```python
from build123d import *

# Parameters (mm, degrees)
SKIZZE1_W                                            = 80
SKIZZE1_H                                            = 120
AUFSATZ_LINEAR_AUSTRAGEN1_DEPTH                      = 5
FORMSENKUNG_F_R_M4_SENKSCHRAUBE_MIT_INNE_D           = 4.3
FORMSENKUNG_F_R_M4_SENKSCHRAUBE_MIT_INNE_DEPTH       = 11.5
FORMSENKUNG_F_R_M4_SENKSCHRAUBE_MIT_INNE_CSINK_D     = 9.18
FORMSENKUNG_F_R_M4_SENKSCHRAUBE_MIT_INNE_CSINK_ANGLE = 90
FORMSENKUNG_F_R_M4_SENKSCHRAUBE_MIT_INNE_TIP         = 1.291850331
F_3_0MM_STIFTLOCH1_D                                 = 3
F_3_0MM_STIFTLOCH1_DEPTH                             = 11.5
F_3_0MM_STIFTLOCH1_TIP                               = 0.901290929
STIRNSENKUNG_F_R_M3_FLACHKOPFSCHRAUB_2_COUNT         = 2
STIRNSENKUNG_F_R_M3_FLACHKOPFSCHRAUB_2_PITCH         = 15
STIRNSENKUNG_F_R_M3_FLACHKOPFSCHRAUB_3_COUNT         = 2
STIRNSENKUNG_F_R_M3_FLACHKOPFSCHRAUB_3_PITCH         = 25
STIRNSENKUNG_F_R_M3_FLACHKOPFSCHRAUB_4_COUNT         = 2
STIRNSENKUNG_F_R_M3_FLACHKOPFSCHRAUB_4_PITCH         = 20
STIRNSENKUNG_F_R_M3_FLACHKOPFSCHRAUB_5_COUNT         = 2
STIRNSENKUNG_F_R_M3_FLACHKOPFSCHRAUB_5_PITCH         = 90
STIRNSENKUNG_F_R_M3_FLACHKOPFSCHRAUB_6_COUNT         = 2
STIRNSENKUNG_F_R_M3_FLACHKOPFSCHRAUB_6_PITCH         = 105
STIRNSENKUNG_F_R_M3_FLACHKOPFSCHRAUB_7_COUNT         = 2
STIRNSENKUNG_F_R_M3_FLACHKOPFSCHRAUB_7_PITCH         = 106.887791632
STIRNSENKUNG_F_R_M3_FLACHKOPFSCHRAUB_8_COUNT         = 2
STIRNSENKUNG_F_R_M3_FLACHKOPFSCHRAUB_8_PITCH         = 92.195444573
M10_GEWINDEBOHRUNG1_D                                = 8.5
LINEARES_MUSTER1_COUNT                               = 2
LINEARES_MUSTER1_PITCH                               = 50


with BuildPart() as part:
    # Skizze1 → Aufsatz-Linear austragen1 (new body)
    with BuildSketch(Plane.XY.offset(10)):
        with Locations((-40, 60)):
            Rectangle(SKIZZE1_W, SKIZZE1_H)
    extrude(amount=-AUFSATZ_LINEAR_AUSTRAGEN1_DEPTH)

    # Formsenkung für M4 Senkschraube mit Innensechskant1
    with Locations(Plane.XY.offset(10)):
        with Locations((-56, 60), (-25, 60)):
            CounterSinkHole(FORMSENKUNG_F_R_M4_SENKSCHRAUBE_MIT_INNE_D / 2, FORMSENKUNG_F_R_M4_SENKSCHRAUBE_MIT_INNE_CSINK_D / 2, depth=FORMSENKUNG_F_R_M4_SENKSCHRAUBE_MIT_INNE_DEPTH, counter_sink_angle=FORMSENKUNG_F_R_M4_SENKSCHRAUBE_MIT_INNE_CSINK_ANGLE)
            with Locations((0, 0, -(FORMSENKUNG_F_R_M4_SENKSCHRAUBE_MIT_INNE_DEPTH + FORMSENKUNG_F_R_M4_SENKSCHRAUBE_MIT_INNE_TIP / 2))):  # 118° drill point
                Cone(0, FORMSENKUNG_F_R_M4_SENKSCHRAUBE_MIT_INNE_D / 2, FORMSENKUNG_F_R_M4_SENKSCHRAUBE_MIT_INNE_TIP, mode=Mode.SUBTRACT)

    # Ø3.0mm Stiftloch1
    with Locations(Plane.XY.offset(10)):
        with Locations((-56, 74), (-25, 74), (-25, 46), (-56, 46)):
            Hole(F_3_0MM_STIFTLOCH1_D / 2, depth=F_3_0MM_STIFTLOCH1_DEPTH)
            with Locations((0, 0, -(F_3_0MM_STIFTLOCH1_DEPTH + F_3_0MM_STIFTLOCH1_TIP / 2))):  # 118° drill point
                Cone(0, F_3_0MM_STIFTLOCH1_D / 2, F_3_0MM_STIFTLOCH1_TIP, mode=Mode.SUBTRACT)

    # Skizze25 → Stirnsenkung für M3 Flachkopfschraube mit Schlitz2 (revolve, cut)
    with BuildSketch(Plane(origin=(-25, 112.5, 5), x_dir=(0, 1, 0), z_dir=(1, 0, 0))):
        Polygon((0, 0), (0, 9.521463052), (1.7, 8.5), (1.7, 2.4), (3.5, 2.4), (3.5, 0), align=None)
    stirnsenkung_f_r_m3_flachkopfschraube_mi = revolve(axis=Axis((-25, 112.5, -1.35), (0, 0, 1)), mode=Mode.SUBTRACT)

    # Stirnsenkung f_r M3 Flachkopfschraub 2: Stirnsenkung für M3 Flachkopfschraube mit Schlitz2 ×2
    with Locations(*[(0, -i * STIRNSENKUNG_F_R_M3_FLACHKOPFSCHRAUB_2_PITCH, 0) for i in range(1, STIRNSENKUNG_F_R_M3_FLACHKOPFSCHRAUB_2_COUNT)]):
        add(stirnsenkung_f_r_m3_flachkopfschraube_mi, mode=Mode.SUBTRACT)

    # Stirnsenkung f_r M3 Flachkopfschraub 3: Stirnsenkung für M3 Flachkopfschraube mit Schlitz2 ×2
    with Locations(*[Vector(0.8000000000000007, -0.5999999999999991, 0) * (i * STIRNSENKUNG_F_R_M3_FLACHKOPFSCHRAUB_3_PITCH) for i in range(1, STIRNSENKUNG_F_R_M3_FLACHKOPFSCHRAUB_3_COUNT)]):
        add(stirnsenkung_f_r_m3_flachkopfschraube_mi, mode=Mode.SUBTRACT)

    # Stirnsenkung f_r M3 Flachkopfschraub 4: Stirnsenkung für M3 Flachkopfschraube mit Schlitz2 ×2
    with Locations(*[(i * STIRNSENKUNG_F_R_M3_FLACHKOPFSCHRAUB_4_PITCH, 0, 0) for i in range(1, STIRNSENKUNG_F_R_M3_FLACHKOPFSCHRAUB_4_COUNT)]):
        add(stirnsenkung_f_r_m3_flachkopfschraube_mi, mode=Mode.SUBTRACT)

    # Stirnsenkung f_r M3 Flachkopfschraub 5: Stirnsenkung für M3 Flachkopfschraube mit Schlitz2 ×2
    with Locations(*[(0, -i * STIRNSENKUNG_F_R_M3_FLACHKOPFSCHRAUB_5_PITCH, 0) for i in range(1, STIRNSENKUNG_F_R_M3_FLACHKOPFSCHRAUB_5_COUNT)]):
        add(stirnsenkung_f_r_m3_flachkopfschraube_mi, mode=Mode.SUBTRACT)

    # Stirnsenkung f_r M3 Flachkopfschraub 6: Stirnsenkung für M3 Flachkopfschraube mit Schlitz2 ×2
    with Locations(*[(0, -i * STIRNSENKUNG_F_R_M3_FLACHKOPFSCHRAUB_6_PITCH, 0) for i in range(1, STIRNSENKUNG_F_R_M3_FLACHKOPFSCHRAUB_6_COUNT)]):
        add(stirnsenkung_f_r_m3_flachkopfschraube_mi, mode=Mode.SUBTRACT)

    # Stirnsenkung f_r M3 Flachkopfschraub 7: Stirnsenkung für M3 Flachkopfschraube mit Schlitz2 ×2
    with Locations(*[Vector(0.1871121078899952, -0.9823385664224747, 0) * (i * STIRNSENKUNG_F_R_M3_FLACHKOPFSCHRAUB_7_PITCH) for i in range(1, STIRNSENKUNG_F_R_M3_FLACHKOPFSCHRAUB_7_COUNT)]):
        add(stirnsenkung_f_r_m3_flachkopfschraube_mi, mode=Mode.SUBTRACT)

    # Stirnsenkung f_r M3 Flachkopfschraub 8: Stirnsenkung für M3 Flachkopfschraube mit Schlitz2 ×2
    with Locations(*[Vector(0.2169304578186558, -0.9761870601839528, 0) * (i * STIRNSENKUNG_F_R_M3_FLACHKOPFSCHRAUB_8_PITCH) for i in range(1, STIRNSENKUNG_F_R_M3_FLACHKOPFSCHRAUB_8_COUNT)]):
        add(stirnsenkung_f_r_m3_flachkopfschraube_mi, mode=Mode.SUBTRACT)

    # M10 Gewindebohrung1 (through all)
    with Locations(Plane(origin=(0, 0, 5), x_dir=(-1, 0, 0), z_dir=(0, 0, -1))):
        with Locations((40, 15)):
            m10_gewindebohrung1 = Hole(M10_GEWINDEBOHRUNG1_D / 2)

    # Lineares Muster1: Stirnsenkung für M3 Flachkopfschraube mit Schlitz2 ×2
    with Locations(*[(-i * LINEARES_MUSTER1_PITCH, 0, 0) for i in range(1, LINEARES_MUSTER1_COUNT)]):
        add(stirnsenkung_f_r_m3_flachkopfschraube_mi, mode=Mode.SUBTRACT)

    # Lineares Muster1 copy 1 sketch → Lineares Muster1 copy 1 (revolve, cut)
    with BuildSketch(Plane(origin=(-75, 97.5, 5), x_dir=(0, 1, 0), z_dir=(1, 0, 0))):
        Polygon((0, 0), (0, 9.521463052), (1.7, 8.5), (1.7, 2.4), (3.5, 2.4), (3.5, 0), align=None)
    revolve(axis=Axis((-75, 97.5, -1.35), (0, 0, 1)), mode=Mode.SUBTRACT)

    # Lineares Muster1 copy 2 sketch → Lineares Muster1 copy 2 (revolve, cut)
    with BuildSketch(Plane(origin=(-55, 97.5, 5), x_dir=(0, 1, 0), z_dir=(1, 0, 0))):
        Polygon((0, 0), (0, 9.521463052), (1.7, 8.5), (1.7, 2.4), (3.5, 2.4), (3.5, 0), align=None)
    revolve(axis=Axis((-55, 97.5, -1.35), (0, 0, 1)), mode=Mode.SUBTRACT)

    # Lineares Muster1 copy 3 sketch → Lineares Muster1 copy 3 (revolve, cut)
    with BuildSketch(Plane(origin=(-55, 112.5, 5), x_dir=(0, 1, 0), z_dir=(1, 0, 0))):
        Polygon((0, 0), (0, 9.521463052), (1.7, 8.5), (1.7, 2.4), (3.5, 2.4), (3.5, 0), align=None)
    revolve(axis=Axis((-55, 112.5, -1.35), (0, 0, 1)), mode=Mode.SUBTRACT)

    # Lineares Muster1 copy 4 sketch → Lineares Muster1 copy 4 (revolve, cut)
    with BuildSketch(Plane(origin=(-75, 22.5, 5), x_dir=(0, 1, 0), z_dir=(1, 0, 0))):
        Polygon((0, 0), (0, 9.521463052), (1.7, 8.5), (1.7, 2.4), (3.5, 2.4), (3.5, 0), align=None)
    revolve(axis=Axis((-75, 22.5, -1.35), (0, 0, 1)), mode=Mode.SUBTRACT)

    # Lineares Muster1 copy 5 sketch → Lineares Muster1 copy 5 (revolve, cut)
    with BuildSketch(Plane(origin=(-75, 7.5, 5), x_dir=(0, 1, 0), z_dir=(1, 0, 0))):
        Polygon((0, 0), (0, 9.521463052), (1.7, 8.5), (1.7, 2.4), (3.5, 2.4), (3.5, 0), align=None)
    revolve(axis=Axis((-75, 7.5, -1.35), (0, 0, 1)), mode=Mode.SUBTRACT)

    # Lineares Muster1 copy 6 sketch → Lineares Muster1 copy 6 (revolve, cut)
    with BuildSketch(Plane(origin=(-55, 7.5, 5), x_dir=(0, 1, 0), z_dir=(1, 0, 0))):
        Polygon((0, 0), (0, 9.521463052), (1.7, 8.5), (1.7, 2.4), (3.5, 2.4), (3.5, 0), align=None)
    revolve(axis=Axis((-55, 7.5, -1.35), (0, 0, 1)), mode=Mode.SUBTRACT)

    # Lineares Muster1 copy 7 sketch → Lineares Muster1 copy 7 (revolve, cut)
    with BuildSketch(Plane(origin=(-55, 22.5, 5), x_dir=(0, 1, 0), z_dir=(1, 0, 0))):
        Polygon((0, 0), (0, 9.521463052), (1.7, 8.5), (1.7, 2.4), (3.5, 2.4), (3.5, 0), align=None)
    revolve(axis=Axis((-55, 22.5, -1.35), (0, 0, 1)), mode=Mode.SUBTRACT)

    # Spiegeln1: M10 Gewindebohrung1 across plane
    add(m10_gewindebohrung1.mirror(Plane(origin=(0, 60, 0), x_dir=(0, 0, 1), z_dir=(0, -1, 0))), mode=Mode.SUBTRACT)


solid = part.part
```
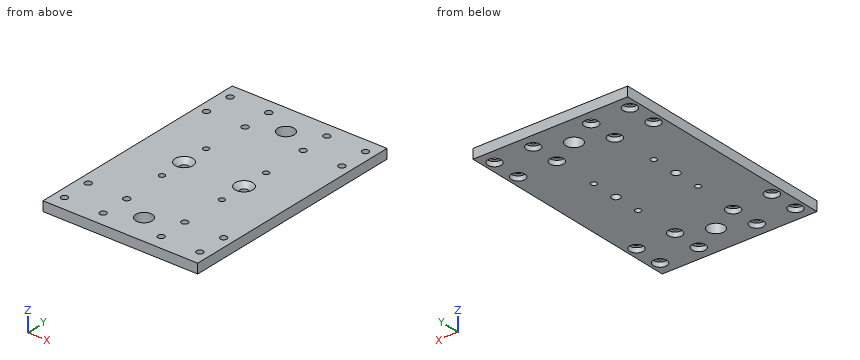
The model under review builds one solid part; all positions refer to its coordinate system, in mm. Round coordinates to 2 decimals unless told otherwise and drop trailing zeros. Write each loop counter-clockwise with the first axis right and the second up, starting at its lowest first coordinate (ties: lowest second). Pieces come first, ordered by that corner, then holes.
(1) We need section D-D on x = -40.5. Give the boundary of the cut face in (y, z).
(2) We need section A-A on y = 74. Give the boundary of the cut face in (x, z).
(3) We need section C-C on y = 105. Give the boundary of the cut face in (x, z), and give its area (4 significant figures).
(4) Insertion check: pin 1 (2.5 mm diameter, centred on x = -55, y = 97.5, fed in from +Z); pin 2 (5.5 mm diameter, centred on x = -25, y = 22.5, fed in from -Z). Each pin has a flat end and moves straight along its axis. Give the tip position at first contact, or say it passes through.
(5) Wall thickness on L1, parallel to Y at x = -75, z = 8.25; L2, parallel to X at y = 22.5, z = 6.2; L3, parallel to Y at x = -75, z = 5.95: over which ranges is each line inside the solid? List them lowest first.
(6) We need section B-B on z = 6.55. Give the number of separate pieces and of enclosed holes in the cut face, and give its area (3 significant figures).
Findings below:
1. outline: (0, 5) - (10.78, 5) - (10.78, 10) - (0, 10) - close; (19.22, 5) - (100.78, 5) - (100.78, 10) - (19.22, 10) - close; (109.22, 5) - (120, 5) - (120, 10) - (109.22, 10) - close
2. outline: (-80, 5) - (-57.5, 5) - (-57.5, 10) - (-80, 10) - close; (-54.5, 5) - (-26.5, 5) - (-26.5, 10) - (-54.5, 10) - close; (-23.5, 5) - (0, 5) - (0, 10) - (-23.5, 10) - close
3. outline: (-80, 5) - (-44.25, 5) - (-44.25, 10) - (-80, 10) - close; (-35.75, 5) - (0, 5) - (0, 10) - (-35.75, 10) - close
3. area: 357.5 mm2
4. pin 1: passes through
4. pin 2: stops at z = 7.4
5. L1: y = 0 to 5.8, 9.2 to 20.8, 24.2 to 95.8, 99.2 to 110.8, 114.2 to 120
5. L2: x = -80 to -78.5, -71.5 to -58.5, -51.5 to -28.5, -21.5 to -8.5, -1.5 to 0
5. L3: y = 0 to 4, 11 to 19, 26 to 94, 101 to 109, 116 to 120
6. separate pieces: 1
6. enclosed holes: 24
6. area: 8,810 mm2
